from build123d import *

# Parameters (mm, degrees)
F0_R     = 0.635
F1_DEPTH = 12.7


# Not quite as in the source:
# - a feature of the source that left no trace in its solid (it failed there, or was rolled back) is left out


with BuildPart() as f1:
    # F0 (on Front) → F1 (new body)
    with BuildSketch(Plane.XZ):
        Polygon((26.5642398671, -2.6142263417), (26.5642398671, 6.35), (-136.7738045981, 6.35), (-136.7738045981, -2.5616034378), (-135.7986113058, -6.3323961114), (-134.0326395944, -6.346404838), (-133.0482363701, -2.54), (-131.0740445981, -2.54), (-130.0892531872, -6.3479058444), (-128.3328795944, -6.3651881602), (-127.3484763701, -2.5587833222), (-125.3742845981, -2.5587833222), (-124.3938092991, -6.35), (-122.6284623376, -6.35), (-121.6487163701, -2.5616034378), (-119.6745245981, -2.5616034378), (-118.6947786306, -6.35), (-116.9287023376, -6.35), (-115.9489563701, -2.5616034378), (-113.9747645981, -2.5616034378), (-112.9899731872, -6.3695092822), (-111.2335995944, -6.3680082758), (-110.2491963701, -2.5616034378), (-108.2750045981, -2.5616034378), (-107.2902131872, -6.3695092822), (-105.5338395944, -6.3680082758), (-104.5494363701, -2.5616034378), (-102.5752445981, -2.5616034378), (-101.5904531872, -6.3695092822), (-99.8340795944, -6.3680082758), (-98.8496763701, -2.5616034378), (-96.8754845981, -2.5616034378), (-95.8906931872, -6.3695092822), (-94.1343195944, -6.3680082758), (-93.1499163701, -2.5616034378), (-91.1757245981, -2.5616034378), (-90.1909331872, -6.3695092822), (-88.4345595944, -6.3680082758), (-87.4501563701, -2.5616034378), (-85.4759645981, -2.5616034378), (-84.4911731872, -6.3695092822), (-82.7347995944, -6.386791598), (-81.7503963701, -2.58038676), (-79.7762045981, -2.58038676), (-78.7914131872, -6.3882926044), (-77.0350395944, -6.3680082758), (-76.0506363701, -2.5616034378), (-74.0764445981, -2.5616034378), (-73.0916531872, -6.3695092822), (-71.3352795944, -6.3680082758), (-70.3508763701, -2.5616034378), (-68.3766845981, -2.5616034378), (-67.3918931872, -6.3695092822), (-65.6355195944, -6.3680082758), (-64.6511163701, -2.5616034378), (-62.6769245981, -2.5616034378), (-61.6921331872, -6.3695092822), (-59.9357595944, -6.3680082758), (-58.9513563701, -2.5616034378), (-56.9771645981, -2.5616034378), (-55.9923731872, -6.3695092822), (-54.2264014758, -6.3835180088), (-53.2419982515, -2.5771131708), (-51.2678064795, -2.5771131708), (-50.2830150686, -6.3850190153), (-48.5266414758, -6.402301331), (-47.5422382515, -2.595896493), (-45.5680464795, -2.595896493), (-44.5875711805, -6.3871131708), (-42.822224219, -6.3871131708), (-41.8424782515, -2.5987166086), (-39.8682864795, -2.5987166086), (-38.888540512, -6.3871131708), (-37.122464219, -6.3871131708), (-36.1427182515, -2.5987166086), (-34.1685264795, -2.5987166086), (-33.1837350686, -6.4066224531), (-31.4273614758, -6.4051214466), (-30.4429582515, -2.5987166086), (-28.4687664795, -2.5987166086), (-27.4839750686, -6.4066224531), (-25.7276014758, -6.4051214466), (-24.7431982515, -2.5987166086), (-22.7690064795, -2.5987166086), (-21.7842150686, -6.4066224531), (-20.0278414758, -6.4051214466), (-19.0434382515, -2.5987166086), (-17.0692464795, -2.5987166086), (-16.0844550686, -6.4066224531), (-14.3280814758, -6.4051214466), (-13.3436782515, -2.5987166086), (-11.3694864795, -2.5987166086), (-10.3846950686, -6.4066224531), (-8.6283214758, -6.4051214466), (-7.6439182515, -2.5987166086), (-5.6697264795, -2.5987166086), (-4.6849350686, -6.4066224531), (-2.9285614758, -6.4239047688), (-1.9441582515, -2.6174999308), (0.0300335205, -2.6174999308), (1.0148249314, -6.4254057753), (2.7711985242, -6.4051214466), (3.7556017485, -2.5987166086), (5.7297935205, -2.5987166086), (6.7145849314, -6.4066224531), (8.4709585242, -6.4051214466), (9.4553617485, -2.5987166086), (11.4295535205, -2.5987166086), (12.4143449314, -6.4066224531), (14.1707185242, -6.4051214466), (15.1551217485, -2.5987166086), (17.1293135205, -2.5987166086), (18.1141049314, -6.4066224531), (19.8704785242, -6.4051214466), (20.8548817485, -2.5987166086), (22.8290735205, -2.5987166086), (23.8138649314, -6.4066224531), (25.5798366429, -6.4206311797), align=None)
        with Locations((-92.0139178634, 0.0037964069)):
            Circle(F0_R, mode=Mode.SUBTRACT)
        with Locations((-12.2076766565, 0.0037964069)):
            Circle(F0_R, mode=Mode.SUBTRACT)
    extrude(amount=-F1_DEPTH)


solid = f1.part
Geometry: final body of the model. Coordinates: model frame, mm. A direction names the side the tool comes from. Give positions to 0.01 mm unless a question says otherwise; leave off trailing zeros. One line per question, with ' | ' between items. Start each with the question number.
(1) Reachability of faces 1 (the flat face through (-54, 6, 6.35)), 2 (the flat face through (-25.242, 6.261, -4.529)) from +Z, -Z, +X, -X, +Y, -Y: full face, straight path, thin tool, end or side. Return the list, or none.
(2) Ray query, line 1 (X direction, y = 9.25, z = 0); line 2 (Z direction, x = -127, y = 3.25); line 3 (Z direction, x = 19, y = 9.5). Return the intervals inside material, ascending. Write a range as from..to.
(3) Section query A-A on z = -4. Count the separate pieces of the cut face and the enclosed holes in it, then the cut area to 3 significant figures.
(4) Contact query for flat-ended pins moving along their axis: pin 1 (1 mm diameter, centred on x = 4.5, y = 4.5, fed in from -Z); pin 2 (5 mm diameter, centred on x = -44.5, y = 8.5, fed in from -Z); pin 3 (1.6 mm diameter, centred on x = -132, y = 6, fed in from -Z). Output: stop coordinate, or through.
The answers:
1) face 1: +Z, +X, -X, +Y, -Y | face 2: -Z, +Y, -Y
2) line 1: -136.77..-92.65, -91.38..-12.84, -11.57..26.56 | line 2: -2.56..6.35 | line 3: -6.41..6.35
3) separate pieces: 29 | enclosed holes: 0 | area: 1,100 mm2
4) pin 1: z = -2.6 | pin 2: z = -6.39 | pin 3: z = -2.54
